Geometry: final body of the model. Coordinates: model frame, mm. Face numbers are marked on the shaded views. A direction names the side the tool comes from. Round coordinates to 2 decimals unless told otherwise and drop trailing zeros. Write each loop counter-clockwise with the first axis right and the second up, starting at its lowest first coordinate (ties: lowest second). Pieces come first, ordered by that corner, then holes. Notation, with made-up numbers: (88, 14) - (99, 14) arc R26 ccw to (99, 53) - close; hole circle Ø7 at (5, 24). An arc over 180 degrees is marked (long way). Write each question's results on one line, items separated by ' | '.
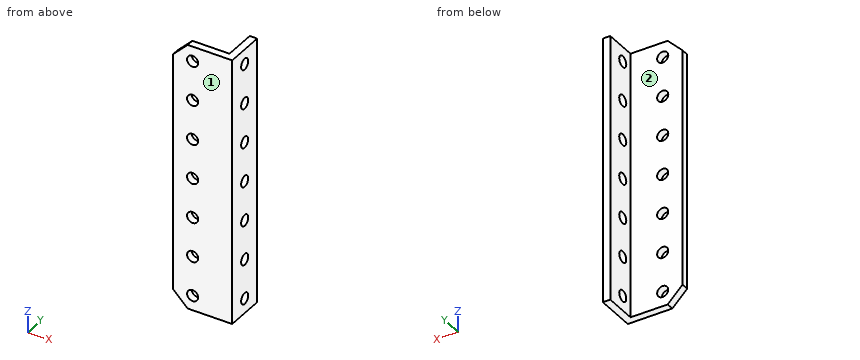
from build123d import *

# Parameters (mm, degrees)
BOSS_EXTRUDE1_DEPTH         = 177.8
F_1_4_CLEARANCE_HOLE1_D     = 7.14248
F_1_4_CLEARANCE_HOLE2_D     = 7.14248
F_1_4_CLEARANCE_HOLE2_DEPTH = 4.7625
CHAMFER1_SIZE               = 12.7
SKETCH10_W                  = 38.1
SKETCH10_H                  = 25.4
CUT_EXTRUDE1_DEPTH          = 3.175


with BuildPart() as part:
    # Sketch1 → Boss-Extrude1 (new body)
    with BuildSketch(Plane.XY):
        Polygon((0, 0), (38.1, 0), (38.1, 25.4), (33.3375, 25.4), (33.3375, 4.7625), (0, 4.7625), align=None)
    extrude(amount=BOSS_EXTRUDE1_DEPTH)

    # 1/4 Clearance Hole1 (through all)
    with Locations(Plane(origin=(0, 4.7625, 0), x_dir=(1, 0, 0), z_dir=(0, 1, 0))):
        with Locations((12.7, -12.7), (12.7, -165.1), (12.7, -139.7), (12.7, -114.3), (12.7, -88.9), (12.7, -63.5), (12.7, -38.1)):
            Hole(F_1_4_CLEARANCE_HOLE1_D / 2)

    # 1/4 Clearance Hole2
    with Locations(Plane.ZY.offset(-33.3375)):
        with Locations((190.5, 12.7), (12.7, 12.7), (38.1, 12.7), (63.5, 12.7), (88.9, 12.7), (114.3, 12.7), (139.7, 12.7), (165.1, 12.7)):
            Hole(F_1_4_CLEARANCE_HOLE2_D / 2, depth=F_1_4_CLEARANCE_HOLE2_DEPTH)

    # Chamfer1
    chamfer1_edges = [part.edges().sort_by_distance(p)[0] for p in [
        (0, 2.38125, 177.8),
        (0, 2.38125, 0),
    ]]
    chamfer(chamfer1_edges, length=CHAMFER1_SIZE)

    # Sketch10 → Cut-Extrude1 (cut)
    with BuildSketch(Plane(origin=(0, 0, 0), x_dir=(-1, 0, 0), z_dir=(0, 0, -1))):
        with Locations((-19.05, 12.7)):
            Rectangle(SKETCH10_W, SKETCH10_H)
    cut_extrude1 = extrude(amount=-CUT_EXTRUDE1_DEPTH, mode=Mode.SUBTRACT)

    # Mirror1: Cut-Extrude1 across plane
    add(cut_extrude1.mirror(Plane(origin=(0, 0, 88.9), x_dir=(1, 0, 0), z_dir=(0, 0, -1))), mode=Mode.SUBTRACT)


solid = part.part
Q1. Section query B-B, the plane y = 12.7. Give the number of separate pieces and of enclosed holes in the cut face, plus the area to 3 significant figures.
Answer block:
separate pieces: 8 | enclosed holes: 0 | area: 578 mm2
Q2. Ray query, line 1 along X through (y, z) = (1.8, 114.3); line 2 along Y through (x, z) = (34.9, 165.1); line 3 along X through (y, z) = (17.5, 82). Return the intervals inside material, ascending.
Answer block:
line 1: 0 to 9.13, 16.27 to 38.1 | line 2: 0 to 9.13, 16.27 to 25.4 | line 3: 33.34 to 38.1
Q3. Section query A-A, the plane x = 36. Return loops of the section in (y, z) (3 decimals).
Answer block:
outline: (0, 3.175) - (25.4, 3.175) - (25.4, 174.625) - (0, 174.625) - close; hole circle Ø7.142 at (12.7, 12.7); hole circle Ø7.142 at (12.7, 38.1); hole circle Ø7.142 at (12.7, 63.5); hole circle Ø7.142 at (12.7, 88.9); hole circle Ø7.142 at (12.7, 114.3); hole circle Ø7.142 at (12.7, 139.7); hole circle Ø7.142 at (12.7, 165.1)
Q4. Section query D-D, the plane z = 38.1. Return loops of the section in (x, y), plus the area to 3 significant figures.
Answer block:
outline: (0, 0) - (9.13, 0) - (9.13, 4.76) - (0, 4.76) - close; (16.27, 0) - (38.1, 0) - (38.1, 9.13) - (33.34, 9.13) - (33.34, 4.76) - (16.27, 4.76) - close; (33.34, 16.27) - (38.1, 16.27) - (38.1, 25.4) - (33.34, 25.4) - close | area: 212 mm2
Q5. Access query for the marked faces 1 and 2. Directions: +Z, -Z, +X, -X, +Y, -Y. A direction counts if a zero-diameter tool reaches every point of the face in a straight line with its end or side. Return the directions, or none.
Answer block:
face 1: +Z, -Z, +X, -X, -Y | face 2: +Z, -Z, -X, +Y
Q6. Pin query (flat end, axial travel): pin 1 (12 mm diameter, centred on x = 7.5, z = 156, fed in from +Y); pin 2 (1 mm diameter, centred on y = 21, z = 43, fed in from -X). Return the tip coordinate at first contact, or that it passes through.
Answer block:
pin 1: y = 4.76 | pin 2: x = 33.34
